CAD build for the part. Positions are in the model's coordinates, mm. A direction names the side the tool comes from. Round coordinates to 2 decimals unless told otherwise and drop trailing zeros. Write each loop counter-clockwise with the first axis right and the second up, starting at its lowest first coordinate (ties: lowest second). Pieces come first, ordered by that corner, then holes. Notation, with made-up numbers: (2.5, 77.5) - (24.5, 77.5) arc R21 cw to (24.5, 114.5) - close; hole circle Ø2 at (9.5, -33.75). An arc over 180 degrees is marked (long way). Put each result on its own line as item: value. Start each with the question number.
Item 1: Drill centre lines: line 1 (Y direction, x = 831.5, z = 459.5); line 2 (X direction, y = 625, z = 598.5). Where is each one in solid material? Low to high. Write a range as from..to.
Item 2: Cut at B-B (z = 373). Give the cut face in (x, y).
Item 3: Mould opens along X. For faces 1 (the flat face through (1038.1, 345, 617)), 2 (the flat face through (0, 706, 296)), 3 (the flat face through (615, 706, 0)) say: released by +X, released by -X, zero draft, split by the parting line, or undercut.
Item 4: Cut at C-C (x = 620). Give the cut face in (y, z), and give its area (3 significant figures).
Item 5: 3-axis set-ups, long thin cutter, end or side, ignore diameter. For faces 4 (the flat face through (1057, 0, 617)), 5 (the flat face through (38.1, 345, 617)), 6 (the flat face through (19, 345, 598.1)): which of +Z, -Z, +X, -X, +Y, -Y reach the whole face in a straight line?
Item 6: Pin check, flat tip, straight feed: pin 1 Ø8 at (x, z) = (564.5, 129) entering from -Y. Stop position of the tip, or through.
Item 7: Cut at A-A (y = 183.5). Give the cut face in (x, z).
```python
from build123d import *

# Parameters (mm, degrees)
CROQUIS1_W                = 38.1
CROQUIS1_H                = 38.1
SALIENTE_EXTRUIR1_DEPTH   = 700
SALIENTE_EXTRUIR1_2_DEPTH = 700
SALIENTE_EXTRUIR1_3_DEPTH = 700
SALIENTE_EXTRUIR1_4_DEPTH = 700
CROQUIS2_W                = 1076.2
CROQUIS2_H                = 636.2
SALIENTE_EXTRUIR2_DEPTH   = 80


with BuildPart() as part:
    # Croquis1 → Saliente-Extruir1 (new body)
    with BuildSketch(Plane(origin=(0, 0, 0), x_dir=(1, 0, 0), z_dir=(0, 1, 0))):
        with Locations((19.05, -19.05)):
            Rectangle(CROQUIS1_W, CROQUIS1_H)
    extrude(amount=SALIENTE_EXTRUIR1_DEPTH)



with BuildPart() as body_2:
    # Croquis1 → Saliente-Extruir1 2 (new body)
    with BuildSketch(Plane(origin=(0, 0, 0), x_dir=(1, 0, 0), z_dir=(0, 1, 0))):
        with Locations((1057.15, -19.05)):
            Rectangle(CROQUIS1_W, CROQUIS1_H)
    extrude(amount=SALIENTE_EXTRUIR1_2_DEPTH)


with BuildPart() as body_3:
    # Croquis1 → Saliente-Extruir1 3 (new body)
    with BuildSketch(Plane(origin=(0, 0, 0), x_dir=(1, 0, 0), z_dir=(0, 1, 0))):
        with Locations((1057.15, -617.15)):
            Rectangle(CROQUIS1_W, CROQUIS1_H)
    extrude(amount=SALIENTE_EXTRUIR1_3_DEPTH)


with BuildPart() as body_4:
    # Croquis1 → Saliente-Extruir1 4 (new body)
    with BuildSketch(Plane(origin=(0, 0, 0), x_dir=(1, 0, 0), z_dir=(0, 1, 0))):
        with Locations((19.05, -617.15)):
            Rectangle(CROQUIS1_W, CROQUIS1_H)
    extrude(amount=SALIENTE_EXTRUIR1_4_DEPTH)


with BuildPart() as part_1:
    add(part.part)

    add(body_2.part)  # Saliente-Extruir2 merges body 2

    add(body_3.part)  # Saliente-Extruir2 merges body 3

    add(body_4.part)  # Saliente-Extruir2 merges body 4
    # Croquis2 → Saliente-Extruir2 (add)
    with BuildSketch(Plane(origin=(0, 700, 0), x_dir=(1, 0, 0), z_dir=(0, 1, 0))):
        with Locations((538.1, -318.1)):
            Rectangle(CROQUIS2_W, CROQUIS2_H)
    extrude(amount=SALIENTE_EXTRUIR2_DEPTH)


solid = part_1.part
```
Output values:
1. line 1: 700..780
1. line 2: 0..38.1, 1038.1..1076.2
2. outline: (0, 700) - (1076.2, 700) - (1076.2, 780) - (0, 780) - close
3. face 1: undercut
3. face 2: released by -X
3. face 3: zero draft
4. outline: (700, 0) - (780, 0) - (780, 636.2) - (700, 636.2) - close
4. area: 50,900 mm2
5. face 4: +Z, -Z, +X, -X, -Y
5. face 5: +Z, -Z, -Y
5. face 6: +X, -X, -Y
6. pin 1: y = 700
7. outline: (0, 0) - (38.1, 0) - (38.1, 38.1) - (0, 38.1) - close; (0, 598.1) - (38.1, 598.1) - (38.1, 636.2) - (0, 636.2) - close; (1038.1, 0) - (1076.2, 0) - (1076.2, 38.1) - (1038.1, 38.1) - close; (1038.1, 598.1) - (1076.2, 598.1) - (1076.2, 636.2) - (1038.1, 636.2) - close
